```python
from build123d import *

# Parameters (mm, degrees)
F0_R     = 5
F1_DEPTH = 25.4
F2_T     = -1
F4_DEPTH = 25.4


with BuildPart() as f1:
    # F0 (on Top) → F1 (new body)
    with BuildSketch(Plane.XY):
        Circle(F0_R)
    extrude(amount=F1_DEPTH)

    # F2
    f2_openings = [f1.faces().sort_by_distance(p)[0] for p in [
        (0, 0, 25.4),
        (0, 0, 0),
    ]]
    offset(amount=F2_T, openings=f2_openings)

    # F3 (on Top) → F4 (cut)
    with BuildSketch(Plane.XY):
        with BuildLine():
            ThreePointArc((4.399024, -2.376676), (4.847428, -1.22574), (5, 0))
            ThreePointArc((5, 0), (4.847428, 1.22574), (4.399024, 2.376676))
            Line((4.399024, 2.376676), (4.399024, -2.376676))
        make_face()
    extrude(amount=F4_DEPTH, mode=Mode.SUBTRACT)


solid = f1.part
```
Model file for the job. Use its own axes, mm. Give positions to 0.01 mm unless a question says otherwise; leave off trailing zeros. Loops run counter-clockwise (first coordinate to the right, second up) from the corner with the lowest first, then second, coordinate; pieces in that order, holes last. Notation, with made-up numbers: (77, 38.5) -> (133, 38.5) arc R20 ccw to (133, 60.5) -> close; hole circle Ø2 at (87, 27.25). An arc over 180 degrees is marked (long way). Use CSV: the item, a comma, the result in double quotes. Start each with the question number.
1) Slice it at B-B on x = 0. Give the cut face in (y, z), plus the area to 3 significant figures.
2) Mould opens along Y. For faces 1 (the cylindrical face through (-5, 0, 13)), 2 (the cylindrical face through (-0.867, -3.905, 12.522)), 3 (the flat face through (-3, 3, 25.4)) say: released by +Y, released by -Y, zero draft, split by the parting line, or undercut.
3) Flat gauge pins, fed straight in: pin 1 Ø1 at (x, z) = (2.5, 9.5) entering from +Y; pin 2 Ø1 at (y, z) = (3.5, 5.5) entering from +X; pin 3 Ø5 at (x, z) = (-3, 18.5) entering from +Y; pin 4 Ø5 at (x, y) = (0, 0) entering from +Z. Where does each tip first touch, or does it go through?
4) Wall check: line 1 (Y direction, x = 0, z = 13.5); line 2 (Y direction, x = 2.75, z = 19.5); line 3 (X direction, y = -2, z = 24.5). Give the ranges that are in metal, low to high.
5) Slice it at A-A on y = 0. Give the cut face in (x, z).
6) Slice it at C-C on z = 5. Give the cut face in (x, y), plus the area to 3 significant figures.
Computed values:
1,outline,"(-5, 0) -> (-4, 0) -> (-4, 25.4) -> (-5, 25.4) -> close; (4, 0) -> (5, 0) -> (5, 25.4) -> (4, 25.4) -> close"
1,area,"50.8 mm^2"
2,face 1,"split by the parting line"
2,face 2,"undercut"
2,face 3,"zero draft"
3,pin 1,"stops at y = 4.58"
3,pin 2,"stops at x = 4"
3,pin 3,"stops at y = 4.97"
3,pin 4,"passes through"
4,line 1,"y = -5 to -4, 4 to 5"
4,line 2,"y = -4.18 to -2.9, 2.9 to 4.18"
4,line 3,"x = -4.58 to -3.46, 3.46 to 4.4"
5,outline,"(-5, 0) -> (-4, 0) -> (-4, 25.4) -> (-5, 25.4) -> close; (4, 0) -> (4.4, 0) -> (4.4, 25.4) -> (4, 25.4) -> close"
6,outline,"(4.4, -2.38) -> (4.4, 2.38) arc R5 ccw (long way) to start; hole circle Ø8 at (0, 0)"
6,area,"26.3 mm^2"
